Model file for the job. Use its own axes, mm. A direction names the side the tool comes from. Coordinates: 2 decimals unless noted, no trailing zeros. Order: outer loops, then holes, each group sorted by start corner. A loop starts at its lowest first (then second) coordinate and runs counter-clockwise, first axis right, second up.
from build123d import *

# Parameters (mm, degrees)
SKETCH_1_R          = 35
SKETCH_1_R_2        = 9.5
EXTRUDE_1_DEPTH     = 18
SKETCH_2_R          = 40.856384021
SKETCH_2_R_2        = 28.650737954
CUT_EXTRUDE_1_DEPTH = 16


with BuildPart() as part:
    # 草图1 → 凸台-拉伸1 (new body)
    with BuildSketch(Plane(origin=(0, 0, 0), x_dir=(1, 0, 0), z_dir=(0, 1, 0))):
        Circle(SKETCH_1_R)
        Circle(SKETCH_1_R_2, mode=Mode.SUBTRACT)
        with BuildLine():
            Line((19.832862473, 17.095228055), (8.333515071, 7.924804513))
            ThreePointArc((8.333515071, 7.924804513), (4.989663, 10.361141981), (1, 11.456439237))
            Line((1, 11.456439237), (1, 26.164656621))
            ThreePointArc((1, 26.164656621), (11.360707431, 23.59075206), (19.832862473, 17.095228055))
        make_face(mode=Mode.SUBTRACT)
        with BuildLine():
            Line((-1, 26.164656621), (-1, 11.456439237))
            ThreePointArc((-1, 11.456439237), (-4.989663, 10.361141981), (-8.333515071, 7.924804513))
            Line((-8.333515071, 7.924804513), (-19.832862473, 17.095228055))
            ThreePointArc((-19.832862473, 17.095228055), (-11.360707431, 23.59075206), (-1, 26.164656621))
        make_face(mode=Mode.SUBTRACT)
        with BuildLine():
            Line((21.079842076, 15.53156509), (9.580494675, 6.361141548))
            ThreePointArc((9.580494675, 6.361141548), (11.21167099, 2.55899074), (11.391723321, -1.574369647))
            Line((11.391723321, -1.574369647), (25.731174987, -4.847255916))
            ThreePointArc((25.731174987, -4.847255916), (25.527277881, 5.826434595), (21.079842076, 15.53156509))
        make_face(mode=Mode.SUBTRACT)
        with BuildLine():
            Line((25.286133119, -6.79711174), (10.946681453, -3.524225471))
            ThreePointArc((10.946681453, -3.524225471), (8.991062048, -7.170132721), (5.871731561, -9.888011351))
            Line((5.871731561, -9.888011351), (12.253387915, -23.139657316))
            ThreePointArc((12.253387915, -23.139657316), (20.471287425, -16.325306958), (25.286133119, -6.79711174))
        make_face(mode=Mode.SUBTRACT)
        with BuildLine():
            Line((10.45145018, -24.007424794), (4.069793825, -10.755778829))
            ThreePointArc((4.069793825, -10.755778829), (0, -11.5), (-4.069793825, -10.755778829))
            Line((-4.069793825, -10.755778829), (-10.45145018, -24.007424794))
            ThreePointArc((-10.45145018, -24.007424794), (0, -26.183759396), (10.45145018, -24.007424794))
        make_face(mode=Mode.SUBTRACT)
        with BuildLine():
            Line((-12.253387915, -23.139657316), (-5.871731561, -9.888011351))
            ThreePointArc((-5.871731561, -9.888011351), (-8.991062048, -7.170132721), (-10.946681453, -3.524225471))
            Line((-10.946681453, -3.524225471), (-25.286133119, -6.79711174))
            ThreePointArc((-25.286133119, -6.79711174), (-20.471287425, -16.325306958), (-12.253387915, -23.139657316))
        make_face(mode=Mode.SUBTRACT)
        with BuildLine():
            Line((-25.731174987, -4.847255916), (-11.391723321, -1.574369647))
            ThreePointArc((-11.391723321, -1.574369647), (-11.21167099, 2.55899074), (-9.580494675, 6.361141548))
            Line((-9.580494675, 6.361141548), (-21.079842076, 15.53156509))
            ThreePointArc((-21.079842076, 15.53156509), (-25.527277881, 5.826434595), (-25.731174987, -4.847255916))
        make_face(mode=Mode.SUBTRACT)
    extrude(amount=EXTRUDE_1_DEPTH)

    # 草图2 → 切除-拉伸1 (cut)
    with BuildSketch(Plane(origin=(0, 18, 0), x_dir=(1, 0, 0), z_dir=(0, 1, 0))):
        Circle(SKETCH_2_R)
        Circle(SKETCH_2_R_2, mode=Mode.SUBTRACT)
    extrude(amount=-CUT_EXTRUDE_1_DEPTH, mode=Mode.SUBTRACT)


solid = part.part
Q1. Cut at D-D, the plane x = -29.5. List the corners of the cut face in (y, z).
Established:
outline: (0, -18.83) - (2, -18.83) - (2, 18.83) - (0, 18.83) - close
Q2. Cut at B-B, the plane z = 0. List the corners of the cut face in (x, y), plus the area to 3 significant figures.
Established:
outline: (-35, 0) - (-26.18, 0) - (-26.18, 18) - (-28.65, 18) - (-28.65, 2) - (-35, 2) - close; (-11.5, 0) - (-9.5, 0) - (-9.5, 18) - (-11.5, 18) - close; (9.5, 0) - (11.5, 0) - (11.5, 18) - (9.5, 18) - close; (26.18, 0) - (35, 0) - (35, 2) - (28.65, 2) - (28.65, 18) - (26.18, 18) - close
area: 186 mm2
Q3. Mould opens along X. For faces 1 (the face through (2, 18, 10)), 2 (the face through (-15.25, 8.87, -10.88)), 3 (the face through (-28, 1, 21)), 4 (the face through (-20.565, 8.874, 16.207)) say: pulls with the +X half, pulls with the -X half, needs draft (parallel to the pull), parting line crosses it, or undercut.
Established:
face 1: needs draft
face 2: undercut
face 3: parting line crosses it
face 4: undercut
Q4. Drop flat-ended pins along their axis: P1, Ø1, axis at x = 3, y = 16, coming from the +Z side; P2, Ø7.5, axis at y = 9.5, z = -18.5, coming from the +X side; P3, Ø8, axis at x = 22.5, y = 2.5, coming from the -Z side. Give the stop position or say it passes through.
Established:
P1: stops at z = 28.54
P2: stops at x = 24.56
P3: stops at z = -29.69
Q5. Cut at A-A, the plane x = 2.5. List the corners of the cut face in (y, z).
Established:
outline: (0, -34.91) - (2, -34.91) - (2, -28.54) - (18, -28.54) - (18, -26.06) - (0, -26.06) - close; (0, -11.22) - (18, -11.22) - (18, -9.17) - (0, -9.17) - close; (0, 9.17) - (18, 9.17) - (18, 11.22) - (0, 11.22) - close; (0, 26.06) - (18, 26.06) - (18, 28.54) - (2, 28.54) - (2, 34.91) - (0, 34.91) - close
Q6. Probe line 1 (X direction, y = 8.5, z = 0); line 2 (X direction, y = 16.5, z = 0.5); line 3 (Z direction, x = 0, y = 9.5). List the from-to ranges inside material, lowest first.
Established:
line 1: x = -28.65 to -26.18, -11.5 to -9.5, 9.5 to 11.5, 26.18 to 28.65
line 2: x = -28.65 to -26.18, -11.49 to -9.49, 9.49 to 11.49, 26.18 to 28.65
line 3: z = -28.65 to -9.5, 9.5 to 11.5, 26.18 to 28.65
Q7. Which spindle directions (+Z, -Z, +X, -X, +Y, -Y) get a long thin tool onto all of the face, cutting with end or side? Do faces 5 (the face through (-25.493, 8.874, -5.973)), 6 (the face through (-29, 2, 0)). Say none if no direction does.
Established:
face 5: +Y, -Y
face 6: +Y
Q8. Cut at C-C, the plane y = 8. Count the separate pieces of the cut face and the enclosed holes in it, plus the area to 3 significant figures.
Established:
separate pieces: 1
enclosed holes: 8
area: 763 mm2
